Build history of the part. All positions in model axes, mm. Face numbers are marked on the shaded views. A direction names the side the tool comes from. Give positions to 0.01 mm unless a question says otherwise; leave off trailing zeros. Order: outer loops, then holes, each group sorted by start corner. A loop starts at its lowest first (then second) coordinate and runs counter-clockwise, first axis right, second up. Notation, with made-up numbers: M -12,15.5 L 5,15.5 A14 cw 5,41.5 Z; hole C -22.5,-25.5 d8. An arc over 180 degrees is marked long. Answer as CSV lines item,"result".
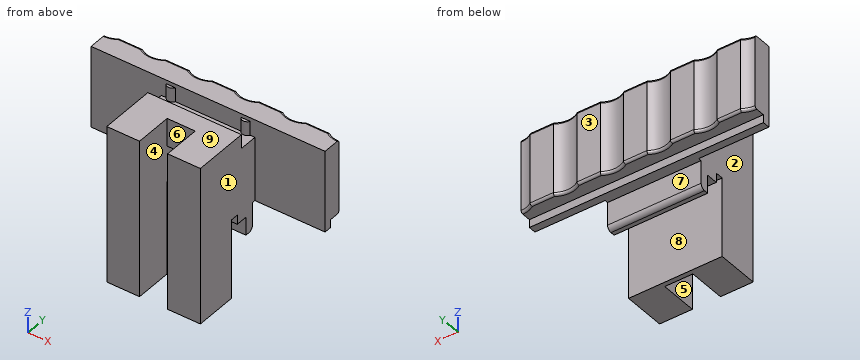
from build123d import *

# Parameters (mm, degrees)
SKETCH1_W            = 25
SKETCH1_H            = 6.85
BOSS_EXTRUDE1_DEPTH  = 0.8
SKETCH2_W            = 10
SKETCH2_H            = 6.85
BOSS_EXTRUDE2_DEPTH  = 3.9
SKETCH3_W            = 3
SKETCH3_H            = 3.85
CUT_EXTRUDE1_DEPTH   = 4.5
BOSS_EXTRUDE3_DEPTH  = 1.5
SKETCH5_W            = 10
SKETCH5_H            = 2.2
BOSS_EXTRUDE4_DEPTH  = 1
SKETCH6_W            = 25
SKETCH6_H            = 0.8
BOSS_EXTRUDE5_DEPTH  = 0.4
SKETCH7_W            = 25
SKETCH7_H            = 7.9
BOSS_EXTRUDE6_DEPTH  = 1.6
SKETCH8_W            = 10
SKETCH8_H            = 0.95
BOSS_EXTRUDE7_DEPTH  = 1.95
SKETCH9_W            = 10
SKETCH9_H            = 0.5
BOSS_EXTRUDE8_DEPTH  = 8.5
SKETCH10_W           = 10
SKETCH10_H           = 1.95
BOSS_EXTRUDE9_DEPTH  = 1.5
SKETCH11_W           = 3.5
SKETCH11_H           = 16.85
BOSS_EXTRUDE10_DEPTH = 4
SKETCH12_W           = 3.5
SKETCH12_H           = 16.85
BOSS_EXTRUDE11_DEPTH = 4
SKETCH13_W           = 2.15
SKETCH13_H           = 7.9
SKETCH14_W           = 7.9
SKETCH14_H           = 2.15
SKETCH15_W           = 2.15
SKETCH15_H           = 7.9
LPATTERN1_COUNT      = 4
LPATTERN1_PITCH      = 5
FILLET1_R            = 0.5
FILLET2_R            = 0.25
FILLET3_R            = 0.25


with BuildPart() as part:
    # Sketch1 → Boss-Extrude1 (new body)
    with BuildSketch(Plane.XZ.offset(4.593725132)):
        with Locations((-3.027595366, 2.575)):
            Rectangle(SKETCH1_W, SKETCH1_H)
    extrude(amount=-BOSS_EXTRUDE1_DEPTH)

    # Sketch2 → Boss-Extrude2 (add)
    with BuildSketch(Plane.XZ.offset(4.593725132)):
        with Locations((-3.027595366, 2.575)):
            Rectangle(SKETCH2_W, SKETCH2_H)
    extrude(amount=BOSS_EXTRUDE2_DEPTH)

    # Sketch3 → Cut-Extrude1 (cut)
    with BuildSketch(Plane.XZ.offset(8.493725132)):
        with Locations((-3.027595366, 2.575)):
            Rectangle(SKETCH3_W, SKETCH3_H)
    extrude(amount=-CUT_EXTRUDE1_DEPTH, mode=Mode.SUBTRACT)

    # Sketch4 → Boss-Extrude3 (add)
    with BuildSketch(Plane.XY.offset(6)):
        with BuildLine():
            Line((0.472404634, -4.593725132), (-6.527595366, -4.593725132))
            ThreePointArc((-6.527595366, -4.593725132), (-7.027595366, -4.890046488), (-7.527595366, -4.593725132))
            Line((-7.527595366, -4.593725132), (-15.527595366, -4.593725132))
            Line((-15.527595366, -4.593725132), (-15.527595366, -3.793725132))
            Line((-15.527595366, -3.793725132), (9.472404634, -3.793725132))
            Line((9.472404634, -3.793725132), (9.472404634, -4.593725132))
            Line((9.472404634, -4.593725132), (1.472404634, -4.593725132))
            ThreePointArc((1.472404634, -4.593725132), (0.972404634, -4.890046488), (0.472404634, -4.593725132))
        make_face()
    extrude(amount=BOSS_EXTRUDE3_DEPTH)

    # Sketch5 → Boss-Extrude4 (add)
    with BuildSketch(Plane(origin=(0, 0, -0.85), x_dir=(-1, 0, 0), z_dir=(0, 0, -1))):
        with Locations((3.027595366, -6.043725132)):
            Rectangle(SKETCH5_W, SKETCH5_H)
    extrude(amount=BOSS_EXTRUDE4_DEPTH)

    # Sketch6 → Boss-Extrude5 (add)
    with BuildSketch(Plane.XY.offset(7.5)):
        with Locations((-3.027595366, -4.193725132)):
            Rectangle(SKETCH6_W, SKETCH6_H)
    extrude(amount=BOSS_EXTRUDE5_DEPTH)

    # Sketch7 → Boss-Extrude6 (add)
    with BuildSketch(Plane(origin=(0, -3.793725132, 0), x_dir=(-1, 0, 0), z_dir=(0, 1, 0))):
        with Locations((3.027595366, 3.95)):
            Rectangle(SKETCH7_W, SKETCH7_H)
    extrude(amount=BOSS_EXTRUDE6_DEPTH)

    # Sketch8 → Boss-Extrude7 (add)
    with BuildSketch(Plane(origin=(0, 0, -1.85), x_dir=(-1, 0, 0), z_dir=(0, 0, -1))):
        with Locations((3.027595366, -5.418725132)):
            Rectangle(SKETCH8_W, SKETCH8_H)
    extrude(amount=BOSS_EXTRUDE7_DEPTH)

    # Sketch9 → Boss-Extrude8 (add)
    with BuildSketch(Plane(origin=(0, 0, -0.85), x_dir=(-1, 0, 0), z_dir=(0, 0, -1))):
        with Locations((3.027595366, -8.243725132)):
            Rectangle(SKETCH9_W, SKETCH9_H)
    extrude(amount=BOSS_EXTRUDE8_DEPTH)

    # Sketch10 → Boss-Extrude9 (add)
    with BuildSketch(Plane.XY.offset(6)):
        with Locations((-3.027595366, -7.518725132)):
            Rectangle(SKETCH10_W, SKETCH10_H)
    extrude(amount=BOSS_EXTRUDE9_DEPTH)

    # Sketch11 → Boss-Extrude10 (add)
    with BuildSketch(Plane.XZ.offset(8.493725132)):
        with Locations((-6.277595366, -0.925)):
            Rectangle(SKETCH11_W, SKETCH11_H)
    extrude(amount=BOSS_EXTRUDE10_DEPTH)

    # Sketch12 → Boss-Extrude11 (add)
    with BuildSketch(Plane.XZ.offset(8.493725132)):
        with Locations((0.222404634, -0.925)):
            Rectangle(SKETCH12_W, SKETCH12_H)
    extrude(amount=BOSS_EXTRUDE11_DEPTH)

    # Sketch13 → Cut-Revolve1 (revolve, cut)
    with BuildSketch(Plane(origin=(-10.497162294, -7.491972288, 0), x_dir=(-0.580930046, 0.813953488, 0), z_dir=(0.813953488, 0.580930046, 0))):
        with Locations((7.584275077, 3.95)):
            Rectangle(SKETCH13_W, SKETCH13_H)
    revolve(axis=Axis((-15.527595366, -0.443725132, 0), (0, 0, 1)), mode=Mode.SUBTRACT)

    # Sketch14 → Cut-Revolve2 (revolve, cut)
    with BuildSketch(Plane(origin=(9.472404634, 0, 0), x_dir=(0, 0, -1), z_dir=(1, 0, 0))):
        with Locations((-3.95, -1.518725132)):
            Rectangle(SKETCH14_W, SKETCH14_H)
    revolve(axis=Axis((9.472404634, -0.443725132, 0), (0, 0, 1)), mode=Mode.SUBTRACT)

    # Sketch15 → Cut-Revolve3 (revolve, cut)
    with BuildSketch(Plane(origin=(-7.184560888, -5.127722099, 0), x_dir=(-0.580930046, 0.813953488, 0), z_dir=(0.813953488, 0.580930046, 0))):
        with Locations((4.679624845, 3.95)):
            Rectangle(SKETCH15_W, SKETCH15_H)
    cut_revolve3 = revolve(axis=Axis((-10.527595366, -0.443725132, 0), (0, 0, 1)), mode=Mode.SUBTRACT)

    # LPattern1: Cut-Revolve3 ×4
    with Locations(*[(i * LPATTERN1_PITCH, 0, 0) for i in range(1, LPATTERN1_COUNT)]):
        add(cut_revolve3, mode=Mode.SUBTRACT)

    # Fillet1
    fillet1_edges = [part.edges().sort_by_distance(p)[0] for p in [
        (-3.027595366, -4.943725132, -3.8),
    ]]
    fillet(fillet1_edges, radius=FILLET1_R)

    # Fillet2
    fillet2_edges = [part.edges().sort_by_distance(p)[0] for p in [
        (-14.871851514, -2.491284655, 0),
        (6.972404634, -2.193725132, 0),
        (8.816660781, -2.491284655, 0),
        (-13.027595366, -2.193725132, 0),
        (-10.527595366, -2.593725132, 0),
        (-8.027595366, -2.193725132, 0),
        (-5.527595366, -2.593725132, 0),
        (-3.027595366, -2.193725132, 0),
        (-0.527595366, -2.593725132, 0),
        (1.972404634, -2.193725132, 0),
        (4.472404634, -2.593725132, 0),
    ]]
    fillet(fillet2_edges, radius=FILLET2_R)

    # Fillet3
    fillet3_edges = [part.edges().sort_by_distance(p)[0] for p in [
        (-13.027595366, -2.193725132, 7.9),
        (-14.871851514, -2.491284655, 7.9),
        (8.816660781, -2.491284655, 7.9),
        (-8.027595366, -2.193725132, 7.9),
        (-10.527595366, -2.593725132, 7.9),
        (-3.027595366, -2.193725132, 7.9),
        (-5.527595366, -2.593725132, 7.9),
        (1.972404634, -2.193725132, 7.9),
        (-0.527595366, -2.593725132, 7.9),
        (6.972404634, -2.193725132, 7.9),
        (4.472404634, -2.593725132, 7.9),
    ]]
    fillet(fillet3_edges, radius=FILLET3_R)


solid = part.part
Item 1: Band-saw the part on A-A (y = -11). Give the cut face in (x, z), and give its area (3 significant figures).
Geometry says:
outline,"M -8.03,-9.35 L -4.53,-9.35 L -4.53,7.5 L -8.03,7.5 Z; M -1.53,-9.35 L 1.97,-9.35 L 1.97,7.5 L -1.53,7.5 Z"
area,"118 mm2"
Item 2: Band-saw the part on D-D (x = -13). Give the cut face in (y, z).
Geometry says:
outline,"M -4.59,-0.85 L -3.79,-0.85 L -3.79,0 L -2.44,0 A0.25 ccw -2.19,0.25 L -2.19,7.65 A0.25 ccw -2.44,7.9 L -4.59,7.9 Z"
Item 3: Pull direction X, two halves, no side cores. Call the marked faces 1, 2, 3 and 4: released by +X, released by -X, zero draft, split by the parting line, or undercut.
Geometry says:
face 1,"released by +X"
face 2,"released by -X"
face 3,"zero draft"
face 4,"undercut"
Item 4: Band-saw the part on B-B (z = 6.5). Give the cut face in (x, y).
Geometry says:
outline,"M -15.53,-4.59 L -7.53,-4.59 A0.57 ccw -6.53,-4.59 L 0.47,-4.59 A0.57 ccw 1.47,-4.59 L 9.47,-4.59 L 9.47,-2.59 A2.15 cw 8.22,-2.19 L 5.72,-2.19 A2.15 cw 3.22,-2.19 L 0.72,-2.19 A2.15 cw -1.78,-2.19 L -4.28,-2.19 A2.15 cw -6.78,-2.19 L -9.28,-2.19 A2.15 cw -11.78,-2.19 L -14.28,-2.19 A2.15 cw -15.53,-2.59 Z; M -8.03,-12.49 L -4.53,-12.49 L -4.53,-8.49 L -1.53,-8.49 L -1.53,-12.49 L 1.97,-12.49 L 1.97,-6.54 L -8.03,-6.54 Z"
Item 5: Band-saw the part on C-C (z = -0.5). Give the cut face in (x, y).
Geometry says:
outline,"M -15.53,-4.59 L -8.03,-4.59 L -8.03,-12.49 L -4.53,-12.49 L -4.53,-8.49 L -1.53,-8.49 L -1.53,-12.49 L 1.97,-12.49 L 1.97,-4.59 L 9.47,-4.59 L 9.47,-3.79 L -15.53,-3.79 Z"
Item 6: Drop flat-ended pins along their axis: pin 1 (0.9 mm diameter, centred on x = -6, z = -0.5, fed in from +Y); pin 2 (5 mm diameter, centred on x = -5.5, y = -11, fed in from +Z); pin 3 (6 mm diameter, centred on y = -8.5, z = 5, fed in from -X). Give the stop position or say it passes through.
Geometry says:
pin 1,"stops at y = -3.79"
pin 2,"stops at z = 7.5"
pin 3,"stops at x = -8.03"
Item 7: 3-axis set-ups, long thin cutter, end or side, ignore diameter. For the marked faces 5, 6, 7, 8 and 9: which of +Z, -Z, +X, -X, +Y, -Y reach the whole face in a straight line?
Geometry says:
face 5,"-Y"
face 6,"+Z, -Z, -Y"
face 7,"-Z, +X, -X, +Y"
face 8,"-Z, +X, -X"
face 9,"+Z, +X, -X, -Y"
Item 8: Probe line 1 along Y through (x, z) = (-5.25, -1.25); line 2 along X through (y, z) = (-10.25, 1.5); line 3 along Y through (x, z) = (-2.75, -2.25). List the from-to ranges inside material, lowest first. Write a range as from..to.
Geometry says:
line 1,"y = -12.49..-7.99, -7.14..-4.94"
line 2,"x = -8.03..-4.53, -1.53..1.97"
line 3,"y = -8.49..-7.99, -5.89..-4.94"
